Geometry check sheet. Reference: drawing and pictorial views, mm from the part's lowest x, y, z. A direction names the side the tool comes from. Round coordinates to 2 decimals unless told otherwise and drop trailing zeros. Write each loop counter-clockwise with the first axis right and the second up, starting at its lowest first coordinate (ties: lowest second). Pieces come first, ordered by that corner, then holes. Notation, with made-up numbers: M 67.25,-23.75 L 93.25,-23.75 A18 cw 93.25,-16.75 Z; hole C -23.5,87.25 d1. An arc over 180 degrees is marked long. One line per item, written item: value. Start each with the question number.
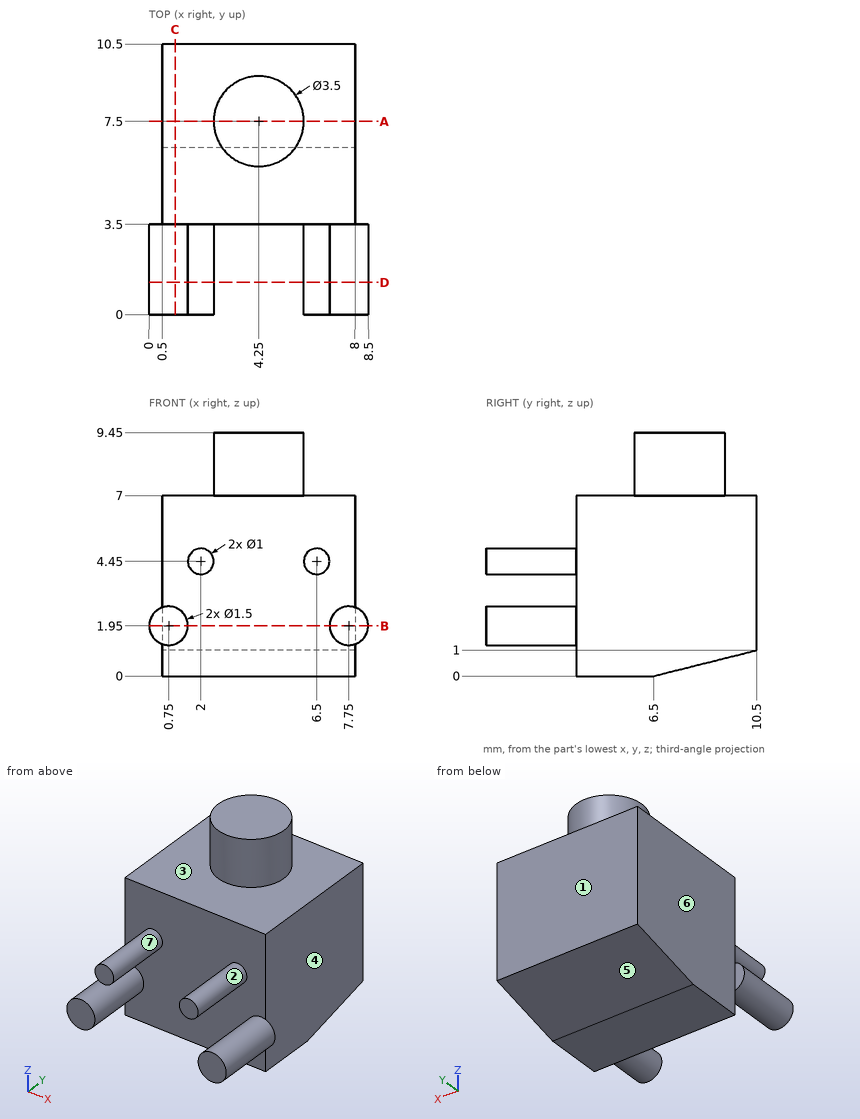
1) Cross-section at A-A (y = 7.5). Record the boundary of the cut face in (x, z).
2) Cross-section at D-D (y = 1.25). Record the boundary of the cut face in (x, z).
3) Thickness scan on line 1 (Y direction, x = 4.5, z = 6.5); line 2 (Z direction, x = 7.75, y = 4); line 3 (X direction, y = 3.75, z = 1.75). Record the ranges inside material, lowest first.
4) Access from +Z, -Z, +X, -X, +Y, -Y to the whole of each face (thin tool, end or side, straight path). Record for the marked faces 1, 2 and 3.
5) Gauge pin test, flat ends, axial feed: pin 1 Ø4 at (y, z) = (5.5, 7.5) entering from +X; pin 2 Ø1 at (x, z) = (3.5, 3.5) entering from -Y; pin 3 Ø0.6 at (x, z) = (8.5, 2) entering from +Y; pin 4 Ø1.5 at (y, z) = (4, 8) entering from -X. Record the tip position at first contact, or that the pin passes through.
6) Cross-section at B-B (z = 1.95). Record the boundary of the cut face in (x, y), then the cut area to 3 significant figures.
7) Mould release check, pull along X, two halves, no side actions. Record for the marked faces 4, 5, 6 and 7: pulls with the +X half, pulls with the -X half, needs draft (parallel to the pull), parting line crosses it, or undercut.
8) Cross-section at C-C (x = 1). Record the boundary of the cut face in (y, z), then the cut area to 3 significant figures.
Results below:
1. outline: M 0.5,0.25 L 8,0.25 L 8,7 L 6,7 L 6,9.45 L 2.5,9.45 L 2.5,7 L 0.5,7 Z
2. outline: C 0.75,1.95 d1.5; C 2,4.45 d1; C 6.5,4.45 d1; C 7.75,1.95 d1.5
3. line 1: y = 3.5 to 10.5
3. line 2: z = 0 to 7
3. line 3: x = 0.5 to 8
4. face 1: +Z, -Z, +X, -X, +Y
4. face 2: -Y
4. face 3: +Z
5. pin 1: stops at x = 8
5. pin 2: stops at y = 3.5
5. pin 3: stops at y = 3.5
5. pin 4: passes through
6. outline: M 0,0 L 1.5,0 L 1.5,3.5 L 7,3.5 L 7,0 L 8.5,0 L 8.5,3.5 L 8,3.5 L 8,10.5 L 0.5,10.5 L 0.5,3.5 L 0,3.5 Z
6. area: 63.0 mm²
7. face 4: pulls with the +X half
7. face 5: needs draft
7. face 6: pulls with the -X half
7. face 7: undercut
8. outline: M 0,1.24 L 3.5,1.24 L 3.5,0 L 6.5,0 L 10.5,1 L 10.5,7 L 3.5,7 L 3.5,2.66 L 0,2.66 Z
8. area: 51.9 mm²
